Can you work these out from the model? Positions are in its coordinate system, mm. Face numbers are marked on the shaded views. A direction names the side the tool comes from. Round coordinates to 2 decimals unless told otherwise and drop trailing zeros. Order: outer loops, then holes, each group sorted by start corner. A loop starts at its lowest first (then second) coordinate and runs counter-clockwise, first axis right, second up. Notation, with made-up numbers: (54, 75.25) -> (81, 75.25) arc R26 ccw to (81, 89.25) -> close; hole circle Ø5 at (17.5, 18). An arc over 180 degrees is marked (long way). One line per item, written item: value.
```python
from build123d import *

# Parameters (mm, degrees)
SKETCH1_R                = 17.5
SKETCH1_R_2              = 4.75
MAINBODY_DEPTH           = 40
SKETCH2_R                = 17.5
SKETCH2_R_2              = 11.25
BEARINGHOUSING_DEPTH     = 7.5
SKETCH3_R                = 1.5
MOUNTINGHOLES_DEPTH      = 20
BOSS_EXTRUDE3_DEPTH      = 40
SKETCH6_R                = 1.5
CUT_EXTRUDE2_DEPTH       = 10
FILLET1_R                = 5
CIRPATTERN1_COUNT        = 6
FILLET1_OF_CIRPATTERN1_R = 5


with BuildPart() as part:
    # Sketch1 → MainBody (new body)
    with BuildSketch(Plane(origin=(0, 0, 0), x_dir=(0, 0, -1), z_dir=(1, 0, 0))):
        Circle(SKETCH1_R)
        Circle(SKETCH1_R_2, mode=Mode.SUBTRACT)
    extrude(amount=MAINBODY_DEPTH)

    # Sketch2 → BearingHousing (add)
    with BuildSketch(Plane(origin=(40, 0, 0), x_dir=(0, 0, -1), z_dir=(1, 0, 0))):
        Circle(SKETCH2_R)
        Circle(SKETCH2_R_2, mode=Mode.SUBTRACT)
    extrude(amount=BEARINGHOUSING_DEPTH)

    # Sketch3 → MountingHoles (cut)
    with BuildSketch(Plane.ZY):
        with Locations((0, 13)):
            Circle(SKETCH3_R)
        with Locations((11.258330249, 6.5)):
            Circle(SKETCH3_R)
        with Locations((11.258330249, -6.5)):
            Circle(SKETCH3_R)
        with Locations((0, -13)):
            Circle(SKETCH3_R)
        with Locations((-11.258330249, -6.5)):
            Circle(SKETCH3_R)
        with Locations((-11.258330249, 6.5)):
            Circle(SKETCH3_R)
    extrude(amount=-MOUNTINGHOLES_DEPTH, mode=Mode.SUBTRACT)

    # Sketch4 → Boss-Extrude3 (add)
    with BuildSketch(Plane.ZY):
        with BuildLine():
            Line((-4.5, 16.911534525), (-4.5, 45))
            Line((-4.5, 45), (-1.7, 45))
            Line((-1.7, 45), (-1.7, 25))
            Line((-1.7, 25), (1.7, 25))
            Line((1.7, 25), (1.7, 45))
            Line((1.7, 45), (4.5, 45))
            Line((4.5, 45), (4.5, 16.911534525))
            ThreePointArc((4.5, 16.911534525), (0, 17.5), (-4.5, 16.911534525))
        make_face()
    boss_extrude3 = extrude(amount=-BOSS_EXTRUDE3_DEPTH)

    # Sketch6 → Cut-Extrude2 (cut)
    with BuildSketch(Plane(origin=(0, 0, -4.5), x_dir=(-1, 0, 0), z_dir=(0, 0, -1))):
        with Locations((-30, 35)):
            Circle(SKETCH6_R)
        with Locations((-20, 35)):
            Circle(SKETCH6_R)
        with Locations((-10, 35)):
            Circle(SKETCH6_R)
    cut_extrude2 = extrude(amount=-CUT_EXTRUDE2_DEPTH, mode=Mode.SUBTRACT)

    # Fillet1
    fillet1_edges = [part.edges().sort_by_distance(p)[0] for p in [
        (20, 16.911534525, 4.5),
        (20, 16.911534525, -4.5),
    ]]
    fillet(fillet1_edges, radius=FILLET1_R)

    # CirPattern1: Boss-Extrude3, Cut-Extrude2 ×6 about axis
    cirpattern1_axis = Axis((0, 0, 0), (1, 0, 0))
    add([boss_extrude3.rotate(cirpattern1_axis, i * 360 / CIRPATTERN1_COUNT) for i in range(1, CIRPATTERN1_COUNT)])
    add([cut_extrude2.rotate(cirpattern1_axis, i * 360 / CIRPATTERN1_COUNT) for i in range(1, CIRPATTERN1_COUNT)], mode=Mode.SUBTRACT)

    # Fillet1 of CirPattern1
    fillet1_of_cirpattern1_edges = [part.edges().sort_by_distance(p)[0] for p in [
        (20, 4.558652946, 16.895818516),
        (20, 12.35288158, 12.395818516),
        (20, -12.35288158, 12.395818516),
        (20, -4.558652946, 16.895818516),
        (20, -16.911534525, -4.5),
        (20, -16.911534525, 4.5),
        (20, -4.558652946, -16.895818516),
        (20, -12.35288158, -12.395818516),
        (20, 12.35288158, -12.395818516),
        (20, 4.558652946, -16.895818516),
    ]]
    fillet(fillet1_of_cirpattern1_edges, radius=FILLET1_OF_CIRPATTERN1_R)


solid = part.part
```
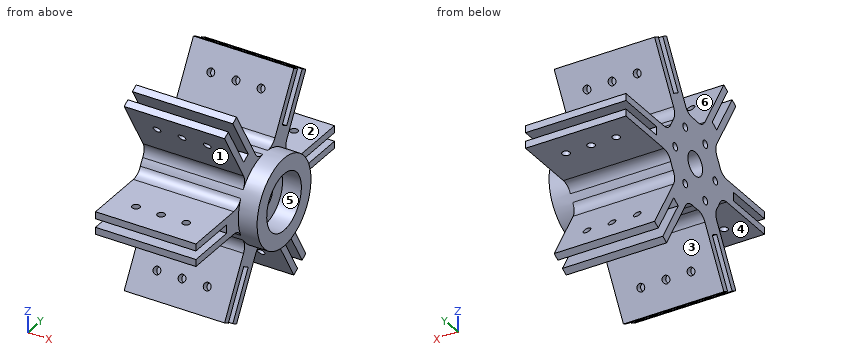
Q1. Will these pins go through, and if not, where does the flat tip stop? pin 1 Ø3.5 at (y, z) = (6.5, 11.26) entering from -X; pin 2 Ø5 at (x, y) = (30, 35) entering from +Z; pin 3 Ø1.5 at (x, z) = (33, 26.5) entering from +Y; pin 4 Ø8.5 at (y, z) = (0, 0) entering from +X.
Answers below:
pin 1: x = 0
pin 2: z = 4.5
pin 3: y = 20.93
pin 4: through
Q2. Please list where these lines run through material, in increasing order: line 1 along X through (y, z) = (-35, -2.65); line 2 along Y through (x, z) = (12.75, 0); line 3 along Z through (x, y) = (15, -0.5).
Answers below:
line 1: 0 to 8.5, 11.5 to 18.5, 21.5 to 28.5, 31.5 to 40
line 2: -25 to -14.5, -11.5 to -4.75, 4.75 to 11.5, 14.5 to 25
line 3: -17.49 to -4.72, 4.72 to 17.49
Q3. We'd pull the mould along Y, two halves only. Please class the marked faces 1, 2 and 3: released by +Y, released by -Y, zero draft, split by the parting line, or undercut.
Answers below:
face 1: released by -Y
face 2: zero draft
face 3: undercut
Q4. On a 3-axis mill with a long thin cutter (end or side, diameter ignored), from which of +Z, -Z, +X, -X, +Y, -Y can I reach the whole of each face in a straight line? I mean the marked faces 4, 5 and 6. Say none if no direction works.
Answers below:
face 4: +X, -X, -Y
face 5: +X
face 6: +Z, +X, -X
Q5. I want a section at A-A on y = 0. List the corners of the cut face in (x, z) for me.
Answers below:
outline: (0, -17.5) -> (47.5, -17.5) -> (47.5, -11.25) -> (40, -11.25) -> (40, -4.75) -> (0, -4.75) -> close; (0, 4.75) -> (40, 4.75) -> (40, 11.25) -> (47.5, 11.25) -> (47.5, 17.5) -> (0, 17.5) -> close
Q6. I want a section at D-D on y = -9.5. List the corners of the cut face in (x, z) for me.
Answers below:
outline: (0, -25.45) -> (40, -25.45) -> (40, -14.7) -> (47.5, -14.7) -> (47.5, -6.03) -> (40, -6.03) -> (40, 6.03) -> (47.5, 6.03) -> (47.5, 14.7) -> (40, 14.7) -> (40, 25.45) -> (0, 25.45) -> close
Q7. I want a section at B-B on x = 30. Give the number of separate pieces and of enclosed holes in the cut face, plus the area to 3 significant figures.
Answers below:
separate pieces: 13
enclosed holes: 1
area: 1,900 mm^2
